Check sheet for the modelled part. Datum: model origin and axes. Units: mm. Face numbers are marked on the shaded views. A direction names the side the tool comes from. Coordinates: 2 decimals unless noted, no trailing zeros. Write each loop counter-clockwise with the first axis right and the second up, starting at its lowest first coordinate (ties: lowest second). Pieces come first, ordered by that corner, then holes. Notation, with made-up numbers: (-16, -9) -> (0, -9) arc R31 ccw to (0, 26) -> close; hole circle Ø7 at (-2.5, 8.5). An arc over 180 degrees is marked (long way). One line per item, written item: value. Start each with the question number.
1) Sectioned sample at A-A on y = 0. Enter the section's corners in (x, z), plus the area to 3 significant figures.
2) Sectioned sample at D-D on z = -10.5. Enter the section's corners in (x, y) (1 decimal).
3) Scan lines: line 1 along Y through (x, z) = (-2, -3.25); line 2 along Z through (x, y) = (-4.25, -1.75); line 3 along Z through (x, y) = (-2.5, -7). Record each from-to range of solid material in increasing order. Write a range as [from, to].
4) Sectioned sample at C-C on z = 0. Enter the section's corners in (x, y) (1 decimal), plus the area to 3 significant figures.
5) Gauge pin test, flat ends, axial feed: P1, Ø1, axis at x = 1, z = 10, coming from the +Y side; P2, Ø8, axis at x = -1.5, z = -6.5, coming from the -Y side; P3, Ø1.5, axis at x = -3.5, z = -10, coming from the +Y side. Record the tip position at first contact, or that the pin passes through.
6) Set-up check for the marked faces 1 and 2: record each of +Z, -Z, +X, -X, +Y, -Y from which the full face is reachable in a straight line by a thin tool's end or side.
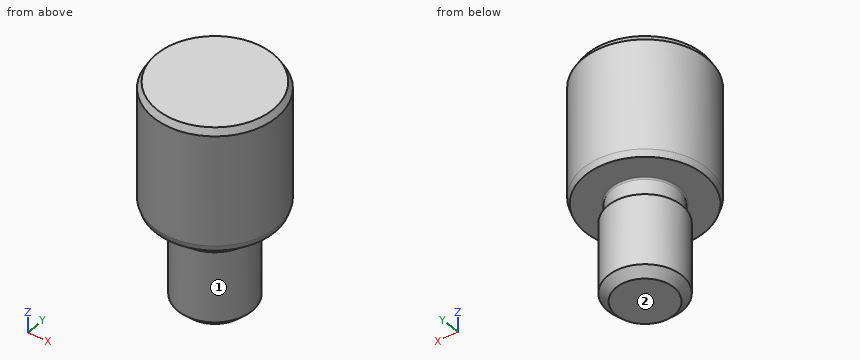
```python
from build123d import *

# Parameters (mm, degrees)
CHAMFER1_SIZE  = 0.809625
CHAMFER1_SIZE2 = 0.467437212
CHAMFER2_SIZE  = 1.04775
FILLET1_R      = 0.1905
CHAMFER4_SIZE  = 0.809625
CHAMFER4_SIZE2 = 0.263063109


with BuildPart() as part:
    # Sketch2 → Revolve2 (revolve)
    with BuildSketch(Plane(origin=(0, 0, 0), x_dir=(0, 0, -1), z_dir=(1, 0, 0)), mode=Mode.PRIVATE) as revolve2_sk:
        Polygon((4.1275, 4.7625), (4.1275, 4.2148125), (3.5798125, 4.2148125), (1.5875, 4.2148125), (1.5875, 7.9375), (-14.2875, 7.9375), (-14.2875, 0), (14.2875, 0), (14.2875, 4.7625), align=None)
    revolve(revolve2_sk.sketch.rotate(Axis((0, 0, 14.2875), (0, 0, -1)), 90), axis=Axis((0, 0, 14.2875), (0, 0, -1)))

    # Chamfer1
    chamfer1_edges = [part.edges().sort_by_distance(p)[0] for p in [
        (-7.9375, 0, 14.2875),
    ]]
    chamfer1_side = [part.faces().sort_by_distance(p)[0] for p in [
        (-7.9375, 0, 6.35),
    ]]
    chamfer(chamfer1_edges, length=CHAMFER1_SIZE, length2=CHAMFER1_SIZE2, reference=chamfer1_side[0])

    # Chamfer2
    chamfer2_edges = [part.edges().sort_by_distance(p)[0] for p in [
        (-4.7625, 0, -14.2875),
    ]]
    chamfer(chamfer2_edges, length=CHAMFER2_SIZE)

    # Fillet1
    fillet1_edges = [part.edges().sort_by_distance(p)[0] for p in [
        (-4.2148125, 0, -1.5875),
    ]]
    fillet(fillet1_edges, radius=FILLET1_R)

    # Chamfer4
    chamfer4_edges = [part.edges().sort_by_distance(p)[0] for p in [
        (-7.9375, 0, -1.5875),
    ]]
    chamfer4_side = [part.faces().sort_by_distance(p)[0] for p in [
        (-7.9375, 0, 5.9451875),
    ]]
    chamfer(chamfer4_edges, length=CHAMFER4_SIZE, length2=CHAMFER4_SIZE2, reference=chamfer4_side[0])


solid = part.part
```
Answers:
1. outline: (-7.94, -0.78) -> (-7.67, -1.59) -> (-4.41, -1.59) arc R0.19 cw to (-4.21, -1.78) -> (-4.21, -4.13) -> (-4.76, -4.13) -> (-4.76, -13.24) -> (-3.71, -14.29) -> (3.71, -14.29) -> (4.76, -13.24) -> (4.76, -4.13) -> (4.21, -4.13) -> (4.21, -1.78) arc R0.19 cw to (4.41, -1.59) -> (7.67, -1.59) -> (7.94, -0.78) -> (7.94, 13.48) -> (7.47, 14.29) -> (-7.47, 14.29) -> (-7.94, 13.48) -> close
1. area: 369 mm2
2. outline: circle Ø9.5 at (0, 0)
3. line 1: y = [-3.71, 3.71]
3. line 2: z = [-13.41, -4.13], [-1.59, 14.29]
3. line 3: z = [-1.59, 14.29]
4. outline: circle Ø15.9 at (0, 0)
4. area: 198 mm2
5. P1: stops at y = 7.92
5. P2: stops at y = -4.76
5. P3: stops at y = 3.89
6. face 1: -Z
6. face 2: -Z, +X, -X, +Y, -Y
